```python
from build123d import *

# Parameters (mm, degrees)
F0_R         = 28.575
F1_DEPTH     = 139.7
F2_T         = -6.35
F5_DEPTH     = 25.4
F7_SIZE      = 6.34999
F8_T4_ANGLE  = 86.6853703019
F8_T11_ANGLE = 86.6853703019


# Not quite as in the source:
# - a fillet or chamfer that OpenCascade refuses, or shapes differently, is made with other operations: its cross-section is extruded or revolved along the edge and cut away or added
# - two fillets or chamfers of one size are made in one step
# - a fillet or chamfer is up to 0.001 mm smaller than in the source, because OpenCascade refuses the exact size


with BuildPart() as f1:
    # F0 (on Top) → F1 (new body)
    with BuildSketch(Plane.XY):
        Circle(F0_R)
    extrude(amount=F1_DEPTH)

    # F2
    f2_openings = [f1.faces().sort_by_distance(p)[0] for p in [
        (0, 0, 139.7),
    ]]
    offset(amount=F2_T, openings=f2_openings)

    # F4 (on offset) → F5 (join)
    with BuildSketch(Plane.XY.offset(114.3)):
        with BuildLine():
            ThreePointArc((10.16, 47.625), (0, 57.785), (-10.16, 47.625))
            ThreePointArc((-10.16, 47.625), (0, 37.465), (10.16, 47.625))
        make_face()
        with BuildLine():
            ThreePointArc((-5.207, 47.625), (0, 52.832), (5.207, 47.625))
            ThreePointArc((5.207, 47.625), (0, 42.418), (-5.207, 47.625))
        make_face(mode=Mode.SUBTRACT)
        with BuildLine():
            ThreePointArc((10.16, 47.625), (0, 37.465), (-10.16, 47.625))
            Line((-10.16, 47.625), (-10.16, 27.305))
            Line((-10.16, 27.305), (10.16, 27.305))
            Line((10.16, 27.305), (10.16, 47.625))
        make_face()
    extrude(amount=-F5_DEPTH)

    # F6: union 

    # F7 (size 6.35 in the source; OpenCascade refuses exactly that, so slightly less here)
    f7_edges = [f1.edges().sort_by_distance(p)[0] for p in [
        (-28.575, 0, 139.7),
    ]]
    chamfer(f7_edges, length=F7_SIZE)

    # F8: chamfer of 5.08 on 3 edges, made by hand


with BuildPart() as f8_tool2:
    # F8_s3 → F8_t4 (revolve)
    with BuildSketch(Plane(origin=(0, 0, 0), x_dir=(0, 0, 1), z_dir=(-0.7272616235, -0.6863603507, 0))):
        Polygon((119.38, 28.575), (114.3, 33.655), (114.3, 28.575), align=None)
    revolve(axis=Axis((0, 0, 114.3), (0, 0, -1)), revolution_arc=F8_T4_ANGLE)

    split(bisect_by=Plane.XZ.offset(-27.305), keep=Keep.BOTTOM)

    split(bisect_by=Plane.YZ.offset(10.16), keep=Keep.BOTTOM)

    split(bisect_by=Plane.YZ.offset(-10.16), keep=Keep.TOP)


with BuildPart() as f1_1:
    add(f1.part)

    # F8_t1: union F8_tool2
    add(f8_tool2.part)


with BuildPart() as f8_tool9:
    # F8_s10 → F8_t11 (revolve)
    with BuildSketch(Plane(origin=(0, 0, 0), x_dir=(0, 0, 1), z_dir=(-0.7272616235, -0.6863603507, 0))):
        Polygon((83.82, 28.575), (88.9, 33.655), (88.9, 28.575), align=None)
    revolve(axis=Axis((0, 0, 88.9), (0, 0, -1)), revolution_arc=F8_T11_ANGLE)

    split(bisect_by=Plane.XZ.offset(-27.305), keep=Keep.BOTTOM)

    split(bisect_by=Plane.YZ.offset(10.16), keep=Keep.BOTTOM)

    split(bisect_by=Plane.YZ.offset(-10.16), keep=Keep.TOP)


with BuildPart() as f1_2:
    add(f1_1.part)

    # F8_t8: union F8_tool9
    add(f8_tool9.part)

    # F8_s15 → F8_t16 (revolve)
    with BuildSketch(Plane.XZ):
        Polygon((22.225, 11.43), (17.145, 6.35), (22.225, 6.35), align=None)
    revolve(axis=Axis((0, 0, 6.35), (0, 0, -1)))


solid = f1_2.part
```
Work out the finished part from the listing and answer in its coordinate system (mm). A direction names the side the tool comes from. Coordinates: 2 decimals unless noted, no trailing zeros. Loops run counter-clockwise (first coordinate to the right, second up) from the corner with the lowest first, then second, coordinate; pieces in that order, holes last.
1) For faces 4 (the flat face through (-10.16, 37, 102)), 5 (the cylindrical face through (0.223, 57.783, 101.778)), 6 (the cylindrical face through (21.199, 6.676, 74.667)), 7 (the conical face through (-0.153, 30.586, 117.369)), 8 (the flat face through (10.16, 37, 102)), determine the directions among +Z, -Z, +X, -X, +Y, -Y from which every point of the face is accessible in a straight line to the end or side of a thin tool.
Results:
face 4: +Z, -Z, -X, +Y
face 5: +Z, -Z, +Y
face 6: +Z
face 7: +Z, +Y
face 8: +Z, -Z, +X, +Y
2) For a pull along Y with two mould halves and no side action, classify faces 1 (the flat face through (0, 0, 6.35)), 2 (the flat face through (0, 42, 114.3)), 3 (the conical face through (-0.153, 30.586, 85.831)) as +Y half, -Y half, draft (parallel to the pull), parting line (faces both ways), or undercut.
Results:
face 1: undercut
face 2: draft
face 3: +Y half
3) Section D-D (z = 36.5) is taken. Give the vertices of the cut face in (x, y) (3 decimals), plus the area to 3 significant figures.
Results:
outline: circle Ø57.15 at (0, 0); hole circle Ø44.45 at (0, 0)
area: 1,010 mm2
4) Consider probe 1 along Y at (x, z) = (0, 104) (3 decimals); probe 2 along X at (y, z) = (-1, 27); probe 3 along Y at (x, z) = (6.5, 32). Determine where each line is inside the solid, lowest interval first.
Results:
probe 1: y = -28.575 to -22.225, 22.225 to 42.418, 52.832 to 57.785
probe 2: x = -28.56 to -22.2, 22.2 to 28.56
probe 3: y = -27.83 to -21.25, 21.25 to 27.83
5) Flat-ended cylindrical pins translate along their axes: pin 1 (8 mm diameter, centred on y = 28.5, z = 74.5, fed in from +X); pin 2 (4 mm diameter, centred on x = 14, y = 32, fed in from +Z); pin 3 (0.9 mm diameter, centred on x = 9, z = 93.5, fed in from -Y); pin 4 (1.5 mm diameter, centred on x = 22.5, y = 9.5, fed in from +Z). Find the tip coordinate at first contact, or state that the pin passes through.
Results:
pin 1: stops at x = 14.71
pin 2: passes through
pin 3: stops at y = -27.27
pin 4: stops at z = 138.25
6) Section B-B (z = 96) is taken. Give the vertices of the cut face in (x, y) (3 decimals).
Results:
outline: (-10.16, 27.305) - (-8.424, 27.305) arc R28.575 ccw (long way) to (8.424, 27.305) - (10.16, 27.305) - (10.16, 47.625) arc R10.16 ccw to (-10.16, 47.625) - close; hole circle Ø44.45 at (0, 0); hole circle Ø10.414 at (0, 47.625)
